Source: CAD feature listing. Evaluate the final solid. Frame: model axes, mm. A direction names the side the tool comes from. Round coordinates to 2 decimals unless told otherwise and drop trailing zeros. Loops run counter-clockwise (first coordinate to the right, second up) from the corner with the lowest first, then second, coordinate; pieces in that order, holes last. Notation, with made-up numbers: M -16.5,24.25 L 8.5,24.25 A35 cw 8.5,62.25 Z; hole C 62.5,-6.5 d5. An arc over 180 degrees is marked long. Answer as a JSON object with one key per item and string values.
Autodesk Fusion 360 part; units mm, degrees
sketch "Sketch3" plane through (0, 0, 0) normal (0, 0, 1) x (1, 0, 0)
  line L0 (-35, 0) -> (35, 0) construction
  line L1 (-35, 7.5) -> (-35, -7.5)
  line L2 (35, 7.5) -> (35, -7.5)
  line L3 (-23, -3.75) -> (23, -3.75)
  line L4 (-23, 3.75) -> (23, 3.75)
  line L5 (0, 3.75) -> (0, -3.75) construction
  line L6 (-35, -7.5) -> (-23, -7.5)
  line L7 (35, -7.5) -> (23, -7.5)
  line L8 (-35, 7.5) -> (-23, 7.5)
  line L9 (-23, 3.75) -> (23, 3.75)
  line L10 (35, 7.5) -> (23, 7.5)
  circle A0 centre (-29, 3.5) radius 1.5
  circle A1 centre (-29, -3.5) radius 1.5
  circle A2 centre (29, 3.5) radius 1.5
  circle A3 centre (29, -3.5) radius 1.5
  line L11 (-29, 3.5) -> (-29, -3.5) construction
  line L12 (29, 3.5) -> (29, -3.5) construction
  line L13 (29, -3.5) -> (-29, -3.5) construction
  line L14 (-29, -3.5) -> (29, 3.5) construction
  line L15 (23, -7.5) -> (23, -3.75)
  line L16 (23, 3.75) -> (23, 7.5)
  line L17 (-23, 7.5) -> (-23, 3.75)
  line L18 (-23, -7.5) -> (-23, -3.75)
  dimension "d9" = 70
  dimension "d10" = 15
  dimension "d13" = 7.5
  dimension "d17" = 3
  dimension "d18" = 3
  dimension "d19" = 3
  dimension "d20" = 3
  dimension "d22" = 7
  dimension "d23" = 7
  dimension "d26" = 6
  dimension "d27" = 12
extrude "Extrude2" add sketch "Sketch3" along normal blind 22
Item 1: Line query: probe 1 along Y at (x, z) = (29, 7.5); probe 2 along X at (y, z) = (-2.75, 10); probe 3 along X at (y, z) = (-4.5, 1.25). Output: solid intervals per line, ascending. Write a range as from..to.
Answer sheet:
{"probe 1": "y = -7.5..-5, -2..2, 5..7.5", "probe 2": "x = -35..-30.3, -27.7..27.7, 30.3..35", "probe 3": "x = -35..-30.12, -27.88..-23, 23..27.88, 30.12..35"}
Item 2: Pull-direction query (Y, two-part tool) for faces 4 (the cylindrical face through (-30.5, 3.43, 10.85)), 5 (the flat face through (0, 0, 22)), 6 (the flat face through (0, 3.75, 11)); classes: pulls with the +Y half, pulls with the -Y half, needs draft (parallel to the pull), parting line crosses it, or undercut.
Answer sheet:
{"face 4": "undercut", "face 5": "needs draft", "face 6": "pulls with the +Y half"}
Item 3: Section A-A on x = -29. Return the cut outline in (y, z).
Answer sheet:
{"outline": "M -7.5,0 L -5,0 L -5,22 L -7.5,22 Z; M -2,0 L 2,0 L 2,22 L -2,22 Z; M 5,0 L 7.5,0 L 7.5,22 L 5,22 Z"}
Item 4: Section B-B on y = 5.75. Return the cut outline in (x, z).
Answer sheet:
{"outline": "M -35,0 L -23,0 L -23,22 L -35,22 Z; M 23,0 L 35,0 L 35,22 L 23,22 Z"}
Item 5: Section C-C on z = 15.25. Return the cut outline in (x, y).
Answer sheet:
{"outline": "M -35,-7.5 L -23,-7.5 L -23,-3.75 L 23,-3.75 L 23,-7.5 L 35,-7.5 L 35,7.5 L 23,7.5 L 23,3.75 L -23,3.75 L -23,7.5 L -35,7.5 Z; hole C -29,-3.5 d3; hole C -29,3.5 d3; hole C 29,-3.5 d3; hole C 29,3.5 d3"}
Item 6: Access query for faces 1 (the flat face through (-23, 6, 11)), 2 (the flat face through (-35, 0, 11)), 3 (the flat face through (-23, -6, 11)). Directions: +Z, -Z, +X, -X, +Y, -Y. A direction counts if a zero-diameter tool reaches every point of the face in a straight line with its end or side. Return the directions, or none.
Answer sheet:
{"face 1": "+Z, -Z, +Y", "face 2": "+Z, -Z, -X, +Y, -Y", "face 3": "+Z, -Z, -Y"}
Item 7: Section D-D on x = 19. Return the cut outline in (y, z), then the cut area to 3 significant figures.
Answer sheet:
{"outline": "M -3.75,0 L 3.75,0 L 3.75,22 L -3.75,22 Z", "area": "165 mm²"}
Item 8: Contact query for flat-ended pins moving along their axis: pin 1 Ø11 at (x, z) = (10.5, 10.5) entering from -Y; pin 2 Ø11 at (x, z) = (10.5, 15.5) entering from +Y. Output: stop coordinate, or through.
Answer sheet:
{"pin 1": "stops at y = -3.75", "pin 2": "stops at y = 3.75"}
